Here's the drawing with two shaded views (mm, measured from the low corner). I have some questions. A direction names the side the tool comes from. Give positions to 0.01 mm unless a question says otherwise; leave off trailing zeros. Write each loop counter-clockwise with the first axis right and the second up, starting at its lowest first coordinate (ties: lowest second). Pieces come first, ordered by that corner, then holes. Notation, with made-up numbers: (80, 2) -> (85, 2) arc R17 cw to (85, 34) -> close; hole circle Ø2 at (85.5, 73.5). An arc over 180 degrees is marked (long way). One line per item, written item: value.
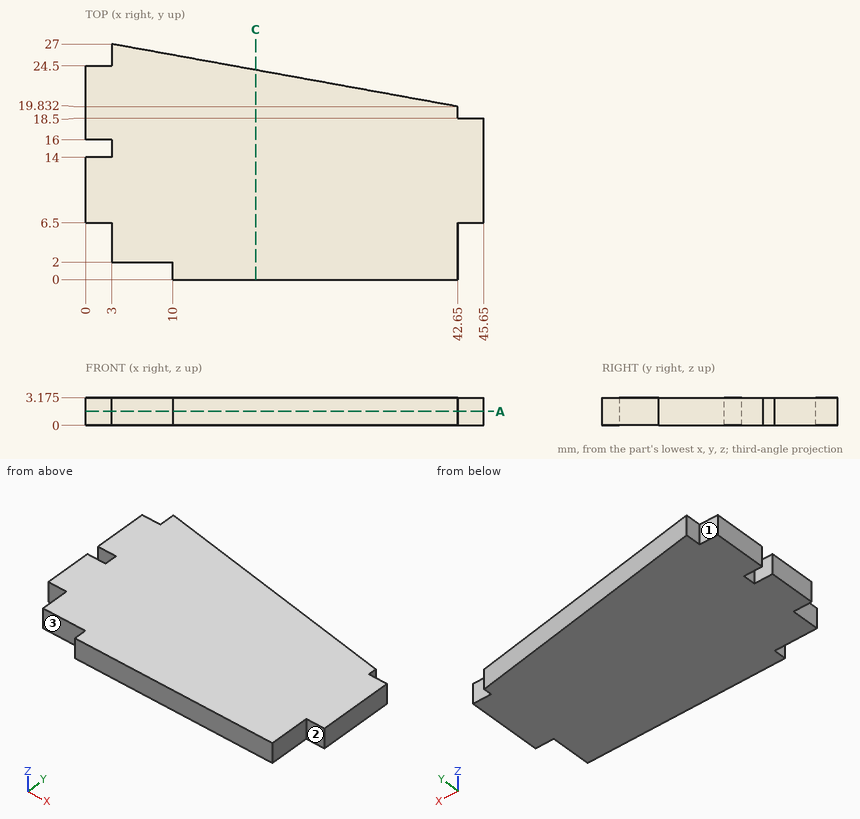
1) Will these pins go through, and if not, where does the flat tip stop? pin 1 (1.5 mm diameter, centred on x = 44.5, z = 1, fed in from +Y); pin 2 (0.9 mm diameter, centred on x = 44, z = 1, fed in from -Y); pin 3 (0.9 mm diameter, centred on x = 2, z = 1.5, fed in from +Y).
Answer list:
pin 1: stops at y = 18.5
pin 2: stops at y = 6.5
pin 3: stops at y = 24.5
2) If we section it at C-C (x = 19.5): Write out the boundary of the cut face in (y, z) (1 decimal).
Answer list:
outline: (0, 0) -> (24, 0) -> (24, 3.2) -> (0, 3.2) -> close
3) If we section it at A-A (z = 1.6): Write out the boundary of the cut face in (x, y).
Answer list:
outline: (0, 6.5) -> (3, 6.5) -> (3, 2) -> (10, 2) -> (10, 0) -> (42.65, 0) -> (42.65, 6.5) -> (45.65, 6.5) -> (45.65, 18.5) -> (42.65, 18.5) -> (42.65, 19.83) -> (3, 27) -> (3, 24.5) -> (0, 24.5) -> (0, 16) -> (3, 16) -> (3, 14) -> (0, 14) -> close
4) For the marked faces 1, 2 and 3, which set-ups out of +Z, -Z, +X, -X, +Y, -Y let a thin tool reach every point of the face, with its end or its side?
Answer list:
face 1: +Z, -Z, -X, +Y
face 2: +Z, -Z, +X, -Y
face 3: +Z, -Z, -X, -Y
5) I need wall thicknesses on L1, parallel to X at y = 2.25, z = 1.45; L2, parallel to Y at x = 19, z = 1.3; L3, parallel to Y at x = 43.5, z = 1.1. Which ranges of each line are inside material? Lowest first, please.
Answer list:
L1: x = 3 to 42.65
L2: y = 0 to 24.11
L3: y = 6.5 to 18.5
